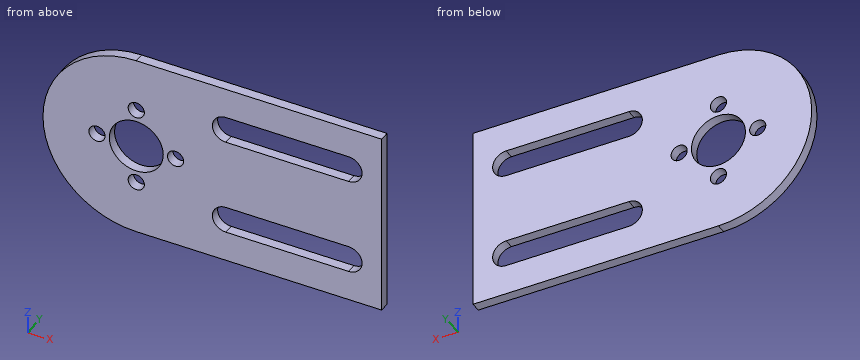
```python
from build123d import *

# Parameters (mm, degrees)
EXTRUDE_1_DEPTH     = 2
SKETCH_2_R          = 5.5
SKETCH_2_R_2        = 1.65
CUT_EXTRUDE_1_DEPTH = 3


with BuildPart() as part:
    # 草图1 → 凸台-拉伸1 (new body)
    with BuildSketch(Plane(origin=(0, 0, 0), x_dir=(1, 0, 0), z_dir=(0, 1, 0))):
        with BuildLine():
            Line((0, 19), (50, 19))
            Line((50, 19), (50, -19))
            Line((50, -19), (0, -19))
            ThreePointArc((0, -19), (-19, 0), (0, 19))
        make_face()
    extrude(amount=EXTRUDE_1_DEPTH)

    # 草图2 → 切除-拉伸1 (cut, through all)
    with BuildSketch(Plane(origin=(0, 2, 0), x_dir=(1, 0, 0), z_dir=(0, 1, 0))):
        Circle(SKETCH_2_R)
        with Locations((0, -8)):
            Circle(SKETCH_2_R_2)
        with Locations((-8, 0)):
            Circle(SKETCH_2_R_2)
        with Locations((0, 8)):
            Circle(SKETCH_2_R_2)
        with Locations((8, 0)):
            Circle(SKETCH_2_R_2)
        with BuildLine():
            Line((18.25, 12.75), (43.25, 12.75))
            ThreePointArc((43.25, 12.75), (46, 10), (43.25, 7.25))
            Line((43.25, 7.25), (18.25, 7.25))
            ThreePointArc((18.25, 7.25), (15.5, 10), (18.25, 12.75))
        make_face()
        with BuildLine():
            Line((43.25, -7.25), (18.25, -7.25))
            ThreePointArc((18.25, -7.25), (15.5, -10), (18.25, -12.75))
            Line((18.25, -12.75), (43.25, -12.75))
            ThreePointArc((43.25, -12.75), (46, -10), (43.25, -7.25))
        make_face()
    extrude(amount=-CUT_EXTRUDE_1_DEPTH, mode=Mode.SUBTRACT)


solid = part.part
```
Can you work these out from the model? Positions are in its coordinate system, mm. Give positions to 0.01 mm unless a question says otherwise; leave off trailing zeros. Order: outer loops, then holes, each group sorted by start corner. A loop starts at its lowest first (then second) coordinate and runs counter-clockwise, first axis right, second up. Notation, with made-up numbers: (17.25, 6.25) - (64.25, 6.25) arc R25 ccw to (64.25, 41.25) - close; hole circle Ø9 at (37, 60.25). An arc over 180 degrees is marked (long way). Use a Markdown table: item, result. Add a question column.
Q1. If we section it at A-A on x = 27: Write out the boundary of the cut face in (y, z), plus the area to 3 significant figures.
Q2. Please list where these lines run through material, in increasing order: line 1 along X through (y, z) = (1.45, 0); line 2 along Z through (x, y) = (18, 1.95); line 3 along Z through (x, y) = (37, 0.85).
Q3. If we section it at D-D on y = 0.7: Write out the boundary of the cut face in (x, z), plus the area to 3 significant figures.
Q4. I'm going to push flat-ended pins straight in: pin 1 (2 mm diameter, centred on x = -8, z = 0, fed in from +Y); pin 2 (1 mm diameter, centred on y = 1.5, z = -9.5, fed in from -X). Where does each tip first touch, or does it pass through?
Q5. If we section it at C-C on z = 1: Write out the boundary of the cut face in (x, y), plus the area to 3 significant figures.
Q6. If we section it at B-B on x = 8: Write out the boundary of the cut face in (y, z), plus the area to 3 significant figures.
Answers follow:
| question | item | result |
|---|---|---|
| 1 | outline | (0, -19) - (2, -19) - (2, -12.75) - (0, -12.75) - close; (0, -7.25) - (2, -7.25) - (2, 7.25) - (0, 7.25) - close; (0, 12.75) - (2, 12.75) - (2, 19) - (0, 19) - close |
| 1 | area | 54.0 mm^2 |
| 2 | line 1 | x = -19 to -9.65, -6.35 to -5.5, 5.5 to 6.35, 9.65 to 50 |
| 2 | line 2 | z = -19 to -12.74, -7.26 to 7.26, 12.74 to 19 |
| 2 | line 3 | z = -19 to -12.75, -7.25 to 7.25, 12.75 to 19 |
| 3 | outline | (0, -19) - (50, -19) - (50, 19) - (0, 19) arc R19 ccw to start; hole circle Ø3.3 at (-8, 0); hole circle Ø11 at (0, 0); hole circle Ø3.3 at (0, -8); hole circle Ø3.3 at (0, 8); hole circle Ø3.3 at (8, 0); hole (18.25, -12.75) - (43.25, -12.75) arc R2.75 ccw to (43.25, -7.25) - (18.25, -7.25) arc R2.75 ccw to start; hole (18.25, 7.25) - (43.25, 7.25) arc R2.75 ccw to (43.25, 12.75) - (18.25, 12.75) arc R2.75 ccw to start |
| 3 | area | 2,020 mm^2 |
| 4 | pin 1 | passes through |
| 4 | pin 2 | stops at x = -16.73 |
| 5 | outline | (-18.97, 0) - (-9.31, 0) - (-9.31, 2) - (-18.97, 2) - close; (-6.69, 0) - (-5.41, 0) - (-5.41, 2) - (-6.69, 2) - close; (5.41, 0) - (6.69, 0) - (6.69, 2) - (5.41, 2) - close; (9.31, 0) - (50, 0) - (50, 2) - (9.31, 2) - close |
| 5 | area | 106 mm^2 |
| 6 | outline | (0, -19) - (2, -19) - (2, -1.65) - (0, -1.65) - close; (0, 1.65) - (2, 1.65) - (2, 19) - (0, 19) - close |
| 6 | area | 69.4 mm^2 |
